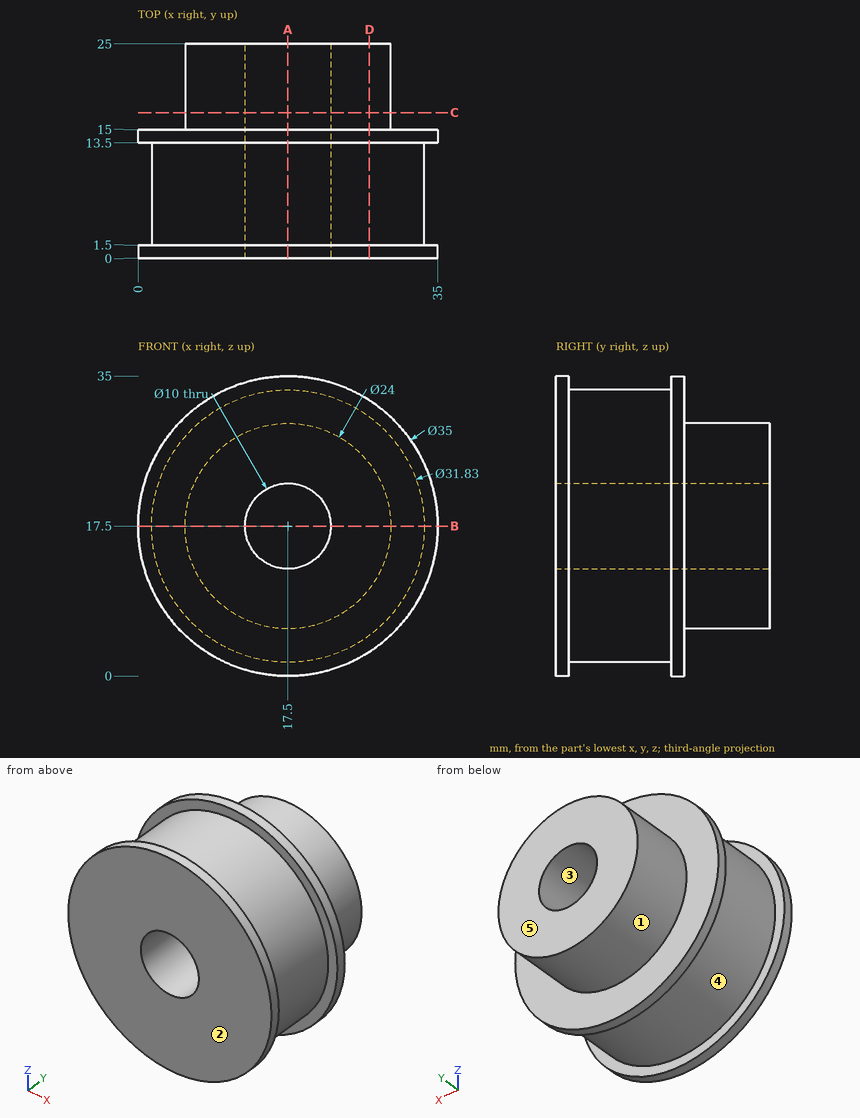
Design review of the part shown in the three views and the two pictorial views. Dimensions are in mm from the part's minimum x, y and z. A direction names the side the tool comes from. Coordinates: 2 decimals unless noted, no trailing zeros. Order: outer loops, then holes, each group sorted by start corner. A loop starts at its lowest first (then second) coordinate and runs counter-clockwise, first axis right, second up.
Item 1: Take a section at A-A, the plane x = 17.5. Write out the cut boundary in (y, z) (3 decimals), then the cut area to 3 significant figures.
Item 2: For the marked faces 1 and 2, list the 3-axis set-ups (+Z, -Z, +X, -X, +Y, -Y) from which the entire face can be reached by the end or side of a thin tool; tool diameter is ignored.
Item 3: Take a section at B-B, the plane z = 17.5. Write out the cut boundary in (x, y) (3 decimals), then the cut area to 3 significant figures.
Item 4: For line 1 (Y direction, x = 29, z = 30.5); line 2 (X direction, y = 5.5, z = 17.5) (3 decimals), list the stretches that pass through material, from the lowest coordinate up.
Item 5: For pin 1 Ø4 at (x, y) = (3.5, 16.5) entering from +Z; pin 2 Ø2 at (x, y) = (13, 6.5) entering from -Z; pin 3 Ø1.5 at (x, z) = (24.5, 4.5) entering from -Y; pin 4 Ø2 at (x, z) = (13.5, 30.5) entering from +Y, all flat-tipped, find the tip position at first contact; note any pin that passes through.
Item 6: The part is to be moulded in two halves that separate along X. For the marked faces 3, 4 and 5, say which applies: pulls with the +X half, pulls with the -X half, needs draft (parallel to the pull), parting line crosses it, or undercut.
Item 7: Take a section at D-D, the plane x = 27. Write out the cut boundary in (y, z), then the cut area to 3 significant figures.
Item 8: Take a section at C-C, the plane y = 17. Write out the cut boundary in (x, z).
The answers:
1. outline: (0, 0) - (1.5, 0) - (1.5, 1.585) - (13.5, 1.585) - (13.5, 0) - (15, 0) - (15, 5.5) - (25, 5.5) - (25, 12.5) - (0, 12.5) - close; (0, 22.5) - (25, 22.5) - (25, 29.5) - (15, 29.5) - (15, 35) - (13.5, 35) - (13.5, 33.415) - (1.5, 33.415) - (1.5, 35) - (0, 35) - close
1. area: 477 mm2
2. face 1: +Y
2. face 2: +Z, -Z, +X, -X, -Y
3. outline: (0, 0) - (12.5, 0) - (12.5, 25) - (5.5, 25) - (5.5, 15) - (0, 15) - (0, 13.5) - (1.585, 13.5) - (1.585, 1.5) - (0, 1.5) - close; (22.5, 0) - (35, 0) - (35, 1.5) - (33.415, 1.5) - (33.415, 13.5) - (35, 13.5) - (35, 15) - (29.5, 15) - (29.5, 25) - (22.5, 25) - close
3. area: 477 mm2
4. line 1: y = 0 to 1.5, 13.5 to 15
4. line 2: x = 1.585 to 12.5, 22.5 to 33.415
5. pin 1: stops at z = 29.56
5. pin 2: stops at z = 1.97
5. pin 3: stops at y = 0
5. pin 4: stops at y = 15
6. face 3: undercut
6. face 4: parting line crosses it
6. face 5: needs draft
7. outline: (0, 2.8) - (1.5, 2.8) - (1.5, 4.73) - (13.5, 4.73) - (13.5, 2.8) - (15, 2.8) - (15, 10.17) - (25, 10.17) - (25, 24.83) - (15, 24.83) - (15, 32.2) - (13.5, 32.2) - (13.5, 30.27) - (1.5, 30.27) - (1.5, 32.2) - (0, 32.2) - close
7. area: 541 mm2
8. outline: circle Ø24 at (17.5, 17.5); hole circle Ø10 at (17.5, 17.5)
